from build123d import *

# Parameters (mm, degrees)
F1_DEPTH = 685.8


with BuildPart() as f1:
    # F0 (on Right) → F1 (new body)
    with BuildSketch(Plane.YZ):
        with BuildLine():
            ThreePointArc((0, 3.175), (0.929936, 0.929936), (3.175, 0))
            Line((3.175, 0), (22.225, 0))
            ThreePointArc((22.225, 0), (24.470064, 0.929936), (25.4, 3.175))
            Line((25.4, 3.175), (25.4, 73.025))
            ThreePointArc((25.4, 73.025), (24.470064, 75.270064), (22.225, 76.2))
            Line((22.225, 76.2), (3.175, 76.2))
            ThreePointArc((3.175, 76.2), (0.929936, 75.270064), (0, 73.025))
            Line((0, 73.025), (0, 3.175))
        make_face()
        with BuildLine():
            Line((19.05, 3.175), (6.35, 3.175))
            ThreePointArc((6.35, 3.175), (4.104936, 4.104936), (3.175, 6.35))
            Line((3.175, 6.35), (3.175, 69.85))
            ThreePointArc((3.175, 69.85), (4.104936, 72.095064), (6.35, 73.025))
            Line((6.35, 73.025), (19.05, 73.025))
            ThreePointArc((19.05, 73.025), (21.295064, 72.095064), (22.225, 69.85))
            Line((22.225, 69.85), (22.225, 6.35))
            ThreePointArc((22.225, 6.35), (21.295064, 4.104936), (19.05, 3.175))
        make_face(mode=Mode.SUBTRACT)
    extrude(amount=F1_DEPTH)


solid = f1.part
Check sheet for the modelled part. Datum: model origin and axes. Units: mm. A direction names the side the tool comes from. Give positions to 0.01 mm unless a question says otherwise; leave off trailing zeros. Write each loop counter-clockwise with the first axis right and the second up, starting at its lowest first coordinate (ties: lowest second). Pieces come first, ordered by that corner, then holes. Notation, with made-up numbers: (-34, 62) -> (14, 62) arc R19 cw to (14, 95) -> close; hole circle Ø2 at (-40, 7). An arc over 180 degrees is marked (long way). Use one line per item in the form item = value. Start each with the question number.
1. Go/stop test with a flat-tipped pin: P1, Ø10, axis at y = 5, z = 12.5, coming from the +X side. Record where the tip stops, or that it passes through.
2. Section check B-B (z = 59.5). Record the cut outline in (x, y) (3 decimals).
3. Access from +Z, -Z, +X, -X, +Y, -Y to the whole of each face (thin tool, end or side, straight path). Record for faces 4 (the flat face through (685.8, 2, 35)), 5 (the flat face through (338, 13, 73.025)).
4. Thickness scan on line 1 along Z through (x, y) = (310.5, 15) (3 decimals); line 2 along Y through (x, z) = (257.5, 34) (3 decimals); line 3 along Z through (x, y) = (85, 20.5). Record the ranges inside material, lowest first. Write a range as from..to.
5. Mould release check, pull along Y, two halves, no side actions. Record for faces 1 (the flat face through (338, 22.225, 39)), 2 (the flat face through (338, 25.4, 38)), 3 (the flat face through (338, 13, 76.2)): pulls with the +Y half, pulls with the -Y half, needs draft (parallel to the pull), parting line crosses it, or undercut.
6. Section check A-A (y = 13.25). Record the cut outline in (x, z) (3 decimals), and give its area (3 significant figures).
7. Section check C-C (x = 494). Record the cut outline in (y, z) (3 decimals).
Conclusion:
q1.P1 = 685.8
q2.outline = (0, 0) -> (685.8, 0) -> (685.8, 3.175) -> (0, 3.175) -> close; (0, 22.225) -> (685.8, 22.225) -> (685.8, 25.4) -> (0, 25.4) -> close
q3.face_4 = +Z, -Z, +X, +Y, -Y
q3.face_5 = +X, -X
q4.line_1 = 0..3.175, 73.025..76.2
q4.line_2 = 0..3.175, 22.225..25.4
q4.line_3 = 0..3.53, 72.67..76.2
q5.face_1 = undercut
q5.face_2 = pulls with the +Y half
q5.face_3 = needs draft
q6.outline = (0, 0) -> (685.8, 0) -> (685.8, 3.175) -> (0, 3.175) -> close; (0, 73.025) -> (685.8, 73.025) -> (685.8, 76.2) -> (0, 76.2) -> close
q6.area = 4,350 mm²
q7.outline = (0, 3.175) arc R3.175 ccw to (3.175, 0) -> (22.225, 0) arc R3.175 ccw to (25.4, 3.175) -> (25.4, 73.025) arc R3.175 ccw to (22.225, 76.2) -> (3.175, 76.2) arc R3.175 ccw to (0, 73.025) -> close; hole (3.175, 6.35) arc R3.175 ccw to (6.35, 3.175) -> (19.05, 3.175) arc R3.175 ccw to (22.225, 6.35) -> (22.225, 69.85) arc R3.175 ccw to (19.05, 73.025) -> (6.35, 73.025) arc R3.175 ccw to (3.175, 69.85) -> close
